Work out the finished part from the listing and answer in its coordinate system (mm). Face numbers are marked on the shaded views. Give positions to 0.01 mm unless a question says otherwise; leave off trailing zeros. Write each loop counter-clockwise with the first axis right and the second up, starting at its lowest first coordinate (ties: lowest second). Pieces come first, ordered by that corner, then holes. Notation, with made-up numbers: (46.5, 45.5) - (56.5, 45.5) arc R24 ccw to (56.5, 69.5) - close; hole circle Ø8 at (3, -32.5). An arc over 180 degrees is marked (long way). Write each question's results on one line, items separated by ' | '. Start each with the question number.
from build123d import *

# Parameters (mm, degrees)
SKETCH1_R           = 34.1376
BOSS_EXTRUDE1_DEPTH = 6.35
SKETCH2_R           = 31.0896
CUT_EXTRUDE3_DEPTH  = 3.175
SKETCH3_R           = 6.35
CUT_EXTRUDE4_DEPTH  = 3.175
SKETCH7_R           = 1.778
CUT_EXTRUDE5_DEPTH  = 3.175


with BuildPart() as part:
    # Sketch1 → Boss-Extrude1 (new body)
    with BuildSketch(Plane(origin=(0, 0, 0), x_dir=(1, 0, 0), z_dir=(0, 1, 0))):
        with Locations(Location((0, 0, 0), (0, 0, 270))):
            Circle(SKETCH1_R)
    extrude(amount=BOSS_EXTRUDE1_DEPTH)

    # Sketch2 → Cut-Extrude3 (cut)
    with BuildSketch(Plane(origin=(0, 6.35, 0), x_dir=(1, 0, 0), z_dir=(0, 1, 0))):
        with Locations(Location((0, 0, 0), (0, 0, 270))):
            Circle(SKETCH2_R)
    extrude(amount=-CUT_EXTRUDE3_DEPTH, mode=Mode.SUBTRACT)

    # Sketch3 → Cut-Extrude4 (cut)
    with BuildSketch(Plane(origin=(0, 3.175, 0), x_dir=(1, 0, 0), z_dir=(0, 1, 0))):
        with Locations(Location((0, 0, 0), (0, 0, 270))):
            Circle(SKETCH3_R)
    extrude(amount=-CUT_EXTRUDE4_DEPTH, mode=Mode.SUBTRACT)

    # Sketch7 → Cut-Extrude5 (cut)
    with BuildSketch(Plane(origin=(0, 3.175, 0), x_dir=(1, 0, 0), z_dir=(0, 1, 0))):
        with Locations(Location((0, 25.4, 0), (0, 0, 270))):
            Circle(SKETCH7_R)
        with Locations(Location((-9.720159182, 23.466540126, 0), (0, 0, 270))):
            Circle(SKETCH7_R)
        with Locations(Location((-17.960512242, 17.960512242, 0), (0, 0, 270))):
            Circle(SKETCH7_R)
        with Locations(Location((-23.466540126, 9.720159182, 0), (0, 0, 270))):
            Circle(SKETCH7_R)
        with Locations(Location((-25.4, 0, 0), (0, 0, 270))):
            Circle(SKETCH7_R)
        with Locations(Location((-23.466540126, -9.720159182, 0), (0, 0, 270))):
            Circle(SKETCH7_R)
        with Locations(Location((-17.960512242, -17.960512242, 0), (0, 0, 270))):
            Circle(SKETCH7_R)
        with Locations(Location((-9.720159182, -23.466540126, 0), (0, 0, 270))):
            Circle(SKETCH7_R)
        with Locations(Location((0, -25.4, 0), (0, 0, 270))):
            Circle(SKETCH7_R)
        with Locations(Location((9.720159182, -23.466540126, 0), (0, 0, 270))):
            Circle(SKETCH7_R)
        with Locations(Location((17.960512242, -17.960512242, 0), (0, 0, 270))):
            Circle(SKETCH7_R)
        with Locations(Location((23.466540126, -9.720159182, 0), (0, 0, 270))):
            Circle(SKETCH7_R)
        with Locations(Location((25.4, 0, 0), (0, 0, 270))):
            Circle(SKETCH7_R)
        with Locations(Location((23.466540126, 9.720159182, 0), (0, 0, 270))):
            Circle(SKETCH7_R)
        with Locations(Location((17.960512242, 17.960512242, 0), (0, 0, 270))):
            Circle(SKETCH7_R)
        with Locations(Location((9.720159182, 23.466540126, 0), (0, 0, 270))):
            Circle(SKETCH7_R)
        with Locations(Location((7.290119387, 17.599905094, 0), (0, 0, 270))):
            Circle(SKETCH7_R)
        with Locations(Location((13.470384182, 13.470384182, 0), (0, 0, 270))):
            Circle(SKETCH7_R)
        with Locations(Location((17.599905094, 7.290119387, 0), (0, 0, 270))):
            Circle(SKETCH7_R)
        with Locations(Location((19.05, 0, 0), (0, 0, 270))):
            Circle(SKETCH7_R)
        with Locations(Location((17.599905094, -7.290119387, 0), (0, 0, 270))):
            Circle(SKETCH7_R)
        with Locations(Location((13.470384182, -13.470384182, 0), (0, 0, 270))):
            Circle(SKETCH7_R)
        with Locations(Location((7.290119387, -17.599905094, 0), (0, 0, 270))):
            Circle(SKETCH7_R)
        with Locations(Location((0, -19.05, 0), (0, 0, 270))):
            Circle(SKETCH7_R)
        with Locations(Location((-7.290119387, -17.599905094, 0), (0, 0, 270))):
            Circle(SKETCH7_R)
        with Locations(Location((-13.470384182, -13.470384182, 0), (0, 0, 270))):
            Circle(SKETCH7_R)
        with Locations(Location((-17.599905094, -7.290119387, 0), (0, 0, 270))):
            Circle(SKETCH7_R)
        with Locations(Location((-19.05, 0, 0), (0, 0, 270))):
            Circle(SKETCH7_R)
        with Locations(Location((-17.599905094, 7.290119387, 0), (0, 0, 270))):
            Circle(SKETCH7_R)
        with Locations(Location((-13.470384182, 13.470384182, 0), (0, 0, 270))):
            Circle(SKETCH7_R)
        with Locations(Location((-7.290119387, 17.599905094, 0), (0, 0, 270))):
            Circle(SKETCH7_R)
        with Locations(Location((0, 19.05, 0), (0, 0, 270))):
            Circle(SKETCH7_R)
        with Locations(Location((0, 9.779, 0), (0, 0, 270))):
            Circle(SKETCH7_R)
        with Locations(Location((-6.914797213, 6.914797213, 0), (0, 0, 270))):
            Circle(SKETCH7_R)
        with Locations(Location((-9.779, 0, 0), (0, 0, 270))):
            Circle(SKETCH7_R)
        with Locations(Location((-6.914797213, -6.914797213, 0), (0, 0, 270))):
            Circle(SKETCH7_R)
        with Locations(Location((0, -9.779, 0), (0, 0, 270))):
            Circle(SKETCH7_R)
        with Locations(Location((6.914797213, -6.914797213, 0), (0, 0, 270))):
            Circle(SKETCH7_R)
        with Locations(Location((9.779, 0, 0), (0, 0, 270))):
            Circle(SKETCH7_R)
        with Locations(Location((6.914797213, 6.914797213, 0), (0, 0, 270))):
            Circle(SKETCH7_R)
    extrude(amount=-CUT_EXTRUDE5_DEPTH, mode=Mode.SUBTRACT)


solid = part.part
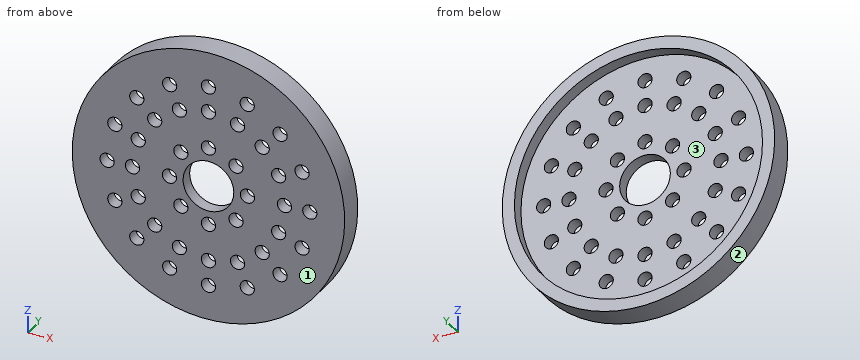
Q1. A cutting plane is placed at D-D, the plane x = -1. Give the number of separate pieces and of enclosed holes in the cut face, and give its area (3 significant figures).
Q2. The mould has two halves that part along X. Classify the marked faces 1, 2 and 3: pulls with the +X half, pulls with the -X half, needs draft (parallel to the pull), parting line crosses it, or undercut.
Q3. A cutting plane is placed at C-C, the plane y = 4.75. Write down the section's boundary in (x, z), and give its area (3 significant figures).
Q4. A cutting plane is placed at B-B, the plane z = 18.5. Write down the section's boundary in (x, y) (3 decimals).
Q5. Consider L1, parallel to X at y = 2, z = -13.5; L2, parallel to X at y = 2.5, z = 14.5; L3, parallel to X at y = 2.5, z = 7. Determine where each line is inside the solid, lowest interval first.
Q6. Given pin 1 (8 mm diameter, centred on x = 23.5, z = 2, fed in from +Y) (3 decimals); pin 2 (2 mm diameter, centred on x = -10, y = 2, fed in from -Z); pin 3 (1.5 mm diameter, centred on x = -7, y = 2.5, fed in from +Z), each flat-ended and moving along its own axis, determine where each tip first touches the part or whether it passes through.
Q7. A cutting plane is placed at A-A, the plane z = 10. Write down the section's boundary in (x, y) (3 decimals), and give its area (3 significant figures).
Result:
1) separate pieces: 8 | enclosed holes: 0 | area: 140 mm2
2) face 1: needs draft | face 2: parting line crosses it | face 3: undercut
3) outline: circle Ø68.28 at (0, 0); hole circle Ø62.18 at (0, 0) | area: 625 mm2
4) outline: (-28.69, 0) - (-19.655, 0) - (-19.655, 3.175) - (-24.986, 3.175) - (-24.986, 6.35) - (-28.69, 6.35) - close; (-16.266, 0) - (-8.823, 0) - (-8.823, 3.175) - (-16.266, 3.175) - close; (-5.757, 0) - (-1.691, 0) - (-1.691, 3.175) - (-5.757, 3.175) - close; (1.691, 0) - (5.757, 0) - (5.757, 3.175) - (1.691, 3.175) - close; (8.823, 0) - (16.266, 0) - (16.266, 3.175) - (8.823, 3.175) - close; (19.655, 0) - (28.69, 0) - (28.69, 6.35) - (24.986, 6.35) - (24.986, 3.175) - (19.655, 3.175) - close
5) L1: x = -31.35 to -15.25, -11.69 to 11.69, 15.25 to 31.35 | L2: x = -30.91 to -14.92, -12.02 to 12.02, 14.92 to 30.91 | L3: x = -33.41 to -19.35, -15.85 to -8.69, -5.14 to 5.14, 8.69 to 15.85, 19.35 to 33.41
6) pin 1: stops at y = 3.175 | pin 2: stops at z = -32.93 | pin 3: stops at z = 33.56
7) outline: (-32.64, 0) - (-25.222, 0) - (-25.222, 3.175) - (-29.437, 3.175) - (-29.437, 6.35) - (-32.64, 6.35) - close; (-21.711, 0) - (-1.764, 0) - (-1.764, 3.175) - (-21.711, 3.175) - close; (1.764, 0) - (21.711, 0) - (21.711, 3.175) - (1.764, 3.175) - close; (25.222, 0) - (32.64, 0) - (32.64, 6.35) - (29.437, 6.35) - (29.437, 3.175) - (25.222, 3.175) - close | area: 194 mm2
